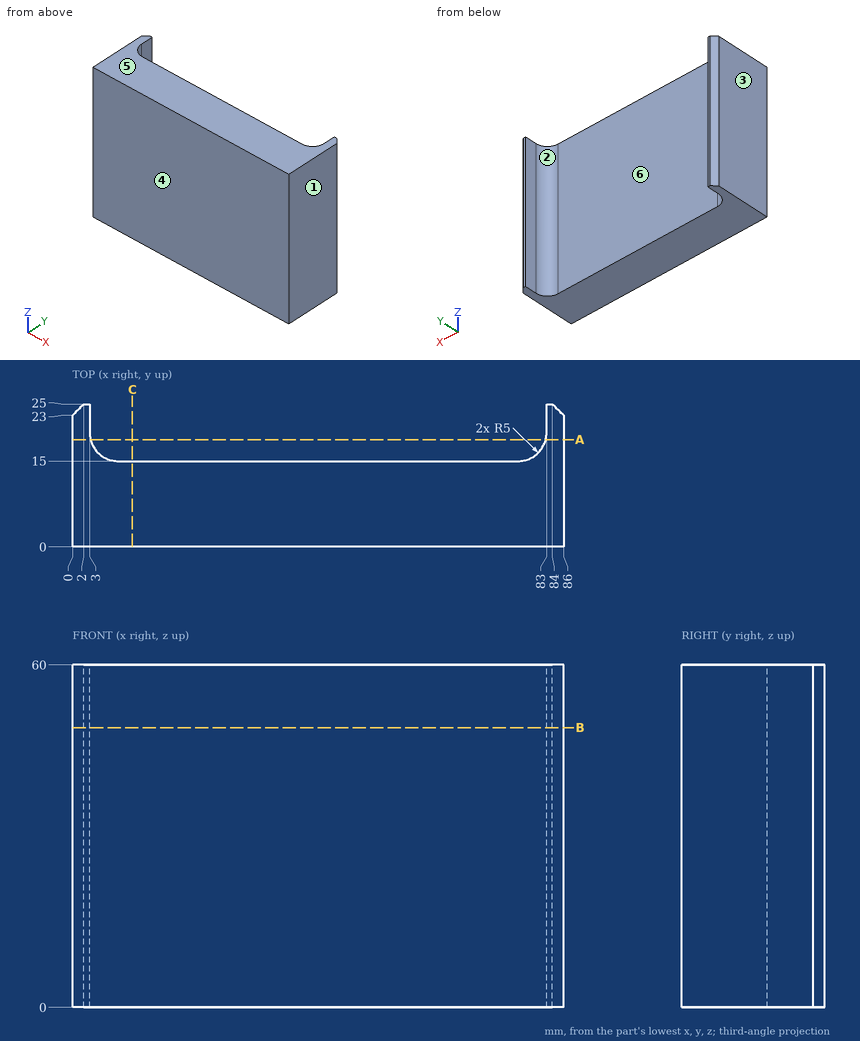
Geometry: see drawing. Coordinates: mm, zero at the bounding-box minimum. A direction names the side the tool comes from. Round coordinates to 2 decimals unless told otherwise and drop trailing zeros. Loops run counter-clockwise (first coordinate to the right, second up) from the corner with the lowest first, then second, coordinate; pieces in that order, holes last.
(1) Section query A-A (y = 18.75). Output: boundary loops of the cut face in (x, z), and give its area (3 significant figures).
From the geometry:
outline: (0, 0) - (3.16, 0) - (3.16, 60) - (0, 60) - close; (82.84, 0) - (86, 0) - (86, 60) - (82.84, 60) - close
area: 379 mm2
(2) Section query B-B (z = 49). Output: boundary loops of the cut face in (x, y), and give its area (3 significant figures).
From the geometry:
outline: (0, 0) - (86, 0) - (86, 23) - (84, 25) - (83, 25) - (83, 20) arc R5 cw to (78, 15) - (8, 15) arc R5 cw to (3, 20) - (3, 25) - (2, 25) - (0, 23) - close
area: 1,360 mm2
(3) Pull-direction query (X, two-part tool) for the marked faces 1, 2, 3 and 4; classes: +X half, -X half, draft (parallel to the pull), parting line (faces both ways), or undercut.
From the geometry:
face 1: +X half
face 2: undercut
face 3: -X half
face 4: draft
(4) Section query C-C (x = 10.5). Output: boundary loops of the cut face in (y, z), and give its area (3 significant figures).
From the geometry:
outline: (0, 0) - (15, 0) - (15, 60) - (0, 60) - close
area: 900 mm2
(5) Material intervals for probe 1 along X at (y, z) = (19.75, 22.5); probe 2 along Y at (x, z) = (52.5, 15); probe 3 along X at (y, z) = (18.5, 50.5), sorted ascending.
From the geometry:
probe 1: x = 0 to 3.01, 82.99 to 86
probe 2: y = 0 to 15
probe 3: x = 0 to 3.23, 82.77 to 86
(6) Access query for the marked faces 5 and 6. Directions: +Z, -Z, +X, -X, +Y, -Y. A direction counts if a zero-diameter tool reaches every point of the face in a straight line with its end or side. Return the directions, or none.
From the geometry:
face 5: +Z, +X, -X, +Y, -Y
face 6: +Z, -Z, +Y
